```python
from build123d import *

# Parameters (mm, degrees)
SKETCH_1_W          = 126.4
SKETCH_1_H          = 68.4
SKETCH_1_W_2        = 124
SKETCH_1_H_2        = 66
EXTRUDE_1_DEPTH     = 40
SKETCH_2_W          = 126.4
SKETCH_2_H          = 68.4
EXTRUDE_1_2_DEPTH   = 1.2
CUT_EXTRUDE_1_DEPTH = 32
CUT_EXTRUDE_2_REACH = 84.243
CUT_EXTRUDE_3_DEPTH = 32
CUT_EXTRUDE_4_REACH = 103.355
CUT_EXTRUDE_5_REACH = 103.355
SKETCH_8_W          = 10
SKETCH_8_H          = 2
SKETCH_8_W_2        = 10.194480457
EXTRUDE_2_DEPTH     = 2
FILLET_1_R          = 2
CUT_EXTRUDE_6_REACH = 139.431
SKETCH_9_W          = 16
SKETCH_9_H          = 1
CUT_EXTRUDE_7_REACH = 104.715
SKETCH_10_W         = 1
SKETCH_10_H         = 16


with BuildPart() as part:
    # Эскиз1 → Extrude 1 (new body)
    with BuildSketch(Plane.XY):
        Rectangle(SKETCH_1_W, SKETCH_1_H)
        Rectangle(SKETCH_1_W_2, SKETCH_1_H_2, mode=Mode.SUBTRACT)
    extrude(amount=EXTRUDE_1_DEPTH)

    # Эскиз2 → Extrude 1 2 (add)
    with BuildSketch(Plane.XY.offset(40)):
        Rectangle(SKETCH_2_W, SKETCH_2_H)
    extrude(amount=-EXTRUDE_1_2_DEPTH)

    # Эскиз3 → Вырез-Вытянуть1 (cut)
    with BuildSketch(Plane.XY.offset(40)):
        with BuildLine():
            Line((59.2, -14), (69.2, -14))
            Line((69.2, -14), (69.2, 14))
            Line((69.2, 14), (59.2, 14))
            ThreePointArc((59.2, 14), (57.785786438, 13.414213562), (57.2, 12))
            Line((57.2, 12), (57.2, -12))
            ThreePointArc((57.2, -12), (57.785786438, -13.414213562), (59.2, -14))
        make_face()
    extrude(amount=-CUT_EXTRUDE_1_DEPTH, mode=Mode.SUBTRACT)

    # Эскиз4 → Вырез-Вытянуть2 (cut, up to next)
    with BuildSketch(Plane.XY.offset(40), mode=Mode.PRIVATE) as cut_extrude_2_sk1:
        with BuildLine():
            Line((51.2, -26), (51.2, 26))
            ThreePointArc((51.2, 26), (53.2, 28), (55.2, 26))
            Line((55.2, 26), (55.2, -26))
            ThreePointArc((55.2, -26), (53.2, -28), (51.2, -26))
        make_face()
    cut_extrude_2_tool1 = extrude(cut_extrude_2_sk1.sketch, amount=-CUT_EXTRUDE_2_REACH, mode=Mode.PRIVATE) & part.part
    # Эскиз4 → Вырез-Вытянуть2 (cut, up to next)
    with BuildSketch(Plane.XY.offset(40), mode=Mode.PRIVATE) as cut_extrude_2_sk2:
        with BuildLine():
            Line((41.2, -26), (41.2, 26))
            ThreePointArc((41.2, 26), (43.2, 28), (45.2, 26))
            Line((45.2, 26), (45.2, -26))
            ThreePointArc((45.2, -26), (43.2, -28), (41.2, -26))
        make_face()
    cut_extrude_2_tool2 = extrude(cut_extrude_2_sk2.sketch, amount=-CUT_EXTRUDE_2_REACH, mode=Mode.PRIVATE) & part.part
    # Эскиз4 → Вырез-Вытянуть2 (cut, up to next)
    with BuildSketch(Plane.XY.offset(40), mode=Mode.PRIVATE) as cut_extrude_2_sk3:
        with BuildLine():
            Line((31.2, -26), (31.2, 26))
            ThreePointArc((31.2, 26), (33.2, 28), (35.2, 26))
            Line((35.2, 26), (35.2, -26))
            ThreePointArc((35.2, -26), (33.2, -28), (31.2, -26))
        make_face()
    cut_extrude_2_tool3 = extrude(cut_extrude_2_sk3.sketch, amount=-CUT_EXTRUDE_2_REACH, mode=Mode.PRIVATE) & part.part
    # Эскиз4 → Вырез-Вытянуть2 (cut, up to next)
    with BuildSketch(Plane.XY.offset(40), mode=Mode.PRIVATE) as cut_extrude_2_sk4:
        with BuildLine():
            Line((21.2, -26), (21.2, 26))
            ThreePointArc((21.2, 26), (23.2, 28), (25.2, 26))
            Line((25.2, 26), (25.2, -26))
            ThreePointArc((25.2, -26), (23.2, -28), (21.2, -26))
        make_face()
    cut_extrude_2_tool4 = extrude(cut_extrude_2_sk4.sketch, amount=-CUT_EXTRUDE_2_REACH, mode=Mode.PRIVATE) & part.part
    # Эскиз4 → Вырез-Вытянуть2 (cut, up to next)
    with BuildSketch(Plane.XY.offset(40), mode=Mode.PRIVATE) as cut_extrude_2_sk5:
        with BuildLine():
            Line((11.2, -26), (11.2, 26))
            ThreePointArc((11.2, 26), (13.2, 28), (15.2, 26))
            Line((15.2, 26), (15.2, -26))
            ThreePointArc((15.2, -26), (13.2, -28), (11.2, -26))
        make_face()
    cut_extrude_2_tool5 = extrude(cut_extrude_2_sk5.sketch, amount=-CUT_EXTRUDE_2_REACH, mode=Mode.PRIVATE) & part.part
    # Эскиз4 → Вырез-Вытянуть2 (cut, up to next)
    with BuildSketch(Plane.XY.offset(40), mode=Mode.PRIVATE) as cut_extrude_2_sk6:
        with BuildLine():
            Line((1.2, -26), (1.2, 26))
            ThreePointArc((1.2, 26), (3.2, 28), (5.2, 26))
            Line((5.2, 26), (5.2, -26))
            ThreePointArc((5.2, -26), (3.2, -28), (1.2, -26))
        make_face()
    cut_extrude_2_tool6 = extrude(cut_extrude_2_sk6.sketch, amount=-CUT_EXTRUDE_2_REACH, mode=Mode.PRIVATE) & part.part
    # Эскиз4 → Вырез-Вытянуть2 (cut, up to next)
    with BuildSketch(Plane.XY.offset(40), mode=Mode.PRIVATE) as cut_extrude_2_sk7:
        with BuildLine():
            Line((-8.8, -26), (-8.8, 26))
            ThreePointArc((-8.8, 26), (-6.8, 28), (-4.8, 26))
            Line((-4.8, 26), (-4.8, -26))
            ThreePointArc((-4.8, -26), (-6.8, -28), (-8.8, -26))
        make_face()
    cut_extrude_2_tool7 = extrude(cut_extrude_2_sk7.sketch, amount=-CUT_EXTRUDE_2_REACH, mode=Mode.PRIVATE) & part.part
    # Эскиз4 → Вырез-Вытянуть2 (cut, up to next)
    with BuildSketch(Plane.XY.offset(40), mode=Mode.PRIVATE) as cut_extrude_2_sk8:
        with BuildLine():
            Line((-18.8, -26), (-18.8, 26))
            ThreePointArc((-18.8, 26), (-16.8, 28), (-14.8, 26))
            Line((-14.8, 26), (-14.8, -26))
            ThreePointArc((-14.8, -26), (-16.8, -28), (-18.8, -26))
        make_face()
    cut_extrude_2_tool8 = extrude(cut_extrude_2_sk8.sketch, amount=-CUT_EXTRUDE_2_REACH, mode=Mode.PRIVATE) & part.part
    # Эскиз4 → Вырез-Вытянуть2 (cut, up to next)
    with BuildSketch(Plane.XY.offset(40), mode=Mode.PRIVATE) as cut_extrude_2_sk9:
        with BuildLine():
            Line((-28.8, -26), (-28.8, 26))
            ThreePointArc((-28.8, 26), (-26.8, 28), (-24.8, 26))
            Line((-24.8, 26), (-24.8, -26))
            ThreePointArc((-24.8, -26), (-26.8, -28), (-28.8, -26))
        make_face()
    cut_extrude_2_tool9 = extrude(cut_extrude_2_sk9.sketch, amount=-CUT_EXTRUDE_2_REACH, mode=Mode.PRIVATE) & part.part
    # Эскиз4 → Вырез-Вытянуть2 (cut, up to next)
    with BuildSketch(Plane.XY.offset(40), mode=Mode.PRIVATE) as cut_extrude_2_sk10:
        with BuildLine():
            Line((-40.127823637, -29.1), (-40.127823637, -5.1))
            ThreePointArc((-40.127823637, -5.1), (-38.127823637, -3.1), (-36.127823637, -5.1))
            Line((-36.127823637, -5.1), (-36.127823637, -29.1))
            ThreePointArc((-36.127823637, -29.1), (-38.127823637, -31.1), (-40.127823637, -29.1))
        make_face()
    cut_extrude_2_tool10 = extrude(cut_extrude_2_sk10.sketch, amount=-CUT_EXTRUDE_2_REACH, mode=Mode.PRIVATE) & part.part
    # Эскиз4 → Вырез-Вытянуть2 (cut, up to next)
    with BuildSketch(Plane.XY.offset(40), mode=Mode.PRIVATE) as cut_extrude_2_sk11:
        with BuildLine():
            Line((-46.127823637, -29.1), (-46.127823637, -5.1))
            ThreePointArc((-46.127823637, -5.1), (-44.127823637, -3.1), (-42.127823637, -5.1))
            Line((-42.127823637, -5.1), (-42.127823637, -29.1))
            ThreePointArc((-42.127823637, -29.1), (-44.127823637, -31.1), (-46.127823637, -29.1))
        make_face()
    cut_extrude_2_tool11 = extrude(cut_extrude_2_sk11.sketch, amount=-CUT_EXTRUDE_2_REACH, mode=Mode.PRIVATE) & part.part
    # Эскиз4 → Вырез-Вытянуть2 (cut, up to next)
    with BuildSketch(Plane.XY.offset(40), mode=Mode.PRIVATE) as cut_extrude_2_sk12:
        with BuildLine():
            Line((-52.127823637, -29.1), (-52.127823637, -5.1))
            ThreePointArc((-52.127823637, -5.1), (-50.127823637, -3.1), (-48.127823637, -5.1))
            Line((-48.127823637, -5.1), (-48.127823637, -29.1))
            ThreePointArc((-48.127823637, -29.1), (-50.127823637, -31.1), (-52.127823637, -29.1))
        make_face()
    cut_extrude_2_tool12 = extrude(cut_extrude_2_sk12.sketch, amount=-CUT_EXTRUDE_2_REACH, mode=Mode.PRIVATE) & part.part
    # Эскиз4 → Вырез-Вытянуть2 (cut, up to next)
    with BuildSketch(Plane.XY.offset(40), mode=Mode.PRIVATE) as cut_extrude_2_sk13:
        with BuildLine():
            Line((-58.127823637, -29.1), (-58.127823637, -5.1))
            ThreePointArc((-58.127823637, -5.1), (-56.127823637, -3.1), (-54.127823637, -5.1))
            Line((-54.127823637, -5.1), (-54.127823637, -29.1))
            ThreePointArc((-54.127823637, -29.1), (-56.127823637, -31.1), (-58.127823637, -29.1))
        make_face()
    cut_extrude_2_tool13 = extrude(cut_extrude_2_sk13.sketch, amount=-CUT_EXTRUDE_2_REACH, mode=Mode.PRIVATE) & part.part
    add(cut_extrude_2_tool1.solids().sort_by_distance((53.2, 0, 40))[0], mode=Mode.SUBTRACT)
    add(cut_extrude_2_tool2.solids().sort_by_distance((43.2, 0, 40))[0], mode=Mode.SUBTRACT)
    add(cut_extrude_2_tool3.solids().sort_by_distance((33.2, 0, 40))[0], mode=Mode.SUBTRACT)
    add(cut_extrude_2_tool4.solids().sort_by_distance((23.2, 0, 40))[0], mode=Mode.SUBTRACT)
    add(cut_extrude_2_tool5.solids().sort_by_distance((13.2, 0, 40))[0], mode=Mode.SUBTRACT)
    add(cut_extrude_2_tool6.solids().sort_by_distance((3.2, 0, 40))[0], mode=Mode.SUBTRACT)
    add(cut_extrude_2_tool7.solids().sort_by_distance((-6.8, 0, 40))[0], mode=Mode.SUBTRACT)
    add(cut_extrude_2_tool8.solids().sort_by_distance((-16.8, 0, 40))[0], mode=Mode.SUBTRACT)
    add(cut_extrude_2_tool9.solids().sort_by_distance((-26.8, 0, 40))[0], mode=Mode.SUBTRACT)
    add(cut_extrude_2_tool10.solids().sort_by_distance((-38.127824, -17.1, 40))[0], mode=Mode.SUBTRACT)
    add(cut_extrude_2_tool11.solids().sort_by_distance((-44.127824, -17.1, 40))[0], mode=Mode.SUBTRACT)
    add(cut_extrude_2_tool12.solids().sort_by_distance((-50.127824, -17.1, 40))[0], mode=Mode.SUBTRACT)
    add(cut_extrude_2_tool13.solids().sort_by_distance((-56.127824, -17.1, 40))[0], mode=Mode.SUBTRACT)

    # Эскиз5 → Вырез-Вытянуть3 (cut)
    with BuildSketch(Plane.XY.offset(40)):
        with BuildLine():
            Line((-59.2, 48.521499027), (-35.2, 48.521499027))
            Line((-35.2, 48.521499027), (-35.2, 21.878500973))
            ThreePointArc((-35.2, 21.878500973), (-35.785786438, 20.46428741), (-37.2, 19.878500973))
            Line((-37.2, 19.878500973), (-57.2, 19.878500973))
            ThreePointArc((-57.2, 19.878500973), (-58.614213562, 20.46428741), (-59.2, 21.878500973))
            Line((-59.2, 21.878500973), (-59.2, 48.521499027))
        make_face()
    extrude(amount=-CUT_EXTRUDE_3_DEPTH, mode=Mode.SUBTRACT)

    # Эскиз6 → Вырез-Вытянуть4 (cut, up to next)
    with BuildSketch(Plane.XZ.offset(34.2), mode=Mode.PRIVATE) as cut_extrude_4_sk1:
        with BuildLine():
            Line((53.2, 0), (-43.2, 0))
            Line((-43.2, 0), (-43.2, 26))
            ThreePointArc((-43.2, 26), (-42.614213562, 27.414213562), (-41.2, 28))
            Line((-41.2, 28), (51.2, 28))
            ThreePointArc((51.2, 28), (52.614213562, 27.414213562), (53.2, 26))
            Line((53.2, 26), (53.2, 0))
        make_face()
    cut_extrude_4_tool1 = extrude(cut_extrude_4_sk1.sketch, amount=-CUT_EXTRUDE_4_REACH, mode=Mode.PRIVATE) & part.part
    add(cut_extrude_4_tool1.solids().sort_by_distance((5, -34.2, 13.991374))[0], mode=Mode.SUBTRACT)

    # Эскиз7 → Вырез-Вытянуть5 (cut, up to next)
    with BuildSketch(Plane(origin=(0, 34.2, 0), x_dir=(1, 0, 0), z_dir=(0, 1, 0)), mode=Mode.PRIVATE) as cut_extrude_5_sk1:
        with BuildLine():
            Line((53.2, 0), (-25.2, 0))
            Line((-25.2, 0), (-25.2, -26))
            ThreePointArc((-25.2, -26), (-24.614213562, -27.414213562), (-23.2, -28))
            Line((-23.2, -28), (51.2, -28))
            ThreePointArc((51.2, -28), (52.614213562, -27.414213562), (53.2, -26))
            Line((53.2, -26), (53.2, 0))
        make_face()
    cut_extrude_5_tool1 = extrude(cut_extrude_5_sk1.sketch, amount=-CUT_EXTRUDE_5_REACH, mode=Mode.PRIVATE) & part.part
    add(cut_extrude_5_tool1.solids().sort_by_distance((14, 34.2, 13.989392))[0], mode=Mode.SUBTRACT)

    # Эскиз8 → Бобышка-Вытянуть2 (add)
    with BuildSketch(Plane(origin=(0, 0, 0), x_dir=(-1, 0, 0), z_dir=(0, 0, -1))):
        with Locations((-58.2, 35.2)):
            Rectangle(SKETCH_8_W, SKETCH_8_H)
        with Locations((-58.2, -35.2)):
            Rectangle(SKETCH_8_W, SKETCH_8_H)
        with Locations((58.102759772, 35.2)):
            Rectangle(SKETCH_8_W_2, SKETCH_8_H)
        with Locations((58.102759772, -35.2)):
            Rectangle(SKETCH_8_W_2, SKETCH_8_H)
    extrude(amount=-EXTRUDE_2_DEPTH)

    # Скругление1
    fillet_1_edges = [part.edges().sort_by_distance(p)[0] for p in [
        (-58.102759771, -34.2, 2),
        (58.2, -34.2, 2),
        (58.2, 34.2, 2),
        (-58.102759771, 34.2, 2),
    ]]
    fillet(fillet_1_edges, radius=FILLET_1_R - 0.0001)  # a hair under: the kernel refuses the full size

    # Эскиз9 → Вырез-Вытянуть6 (cut, up to next)
    with BuildSketch(Plane(origin=(63.2, 0, 0), x_dir=(0, 0, -1), z_dir=(1, 0, 0)), mode=Mode.PRIVATE) as cut_extrude_6_sk1:
        Rectangle(SKETCH_9_W, SKETCH_9_H)
    cut_extrude_6_tool1 = extrude(cut_extrude_6_sk1.sketch, amount=-CUT_EXTRUDE_6_REACH, mode=Mode.PRIVATE) & part.part
    add(cut_extrude_6_tool1.solids().sort_by_distance((63.2, 0, 0))[0], mode=Mode.SUBTRACT)

    # Эскиз10 → Вырез-Вытянуть7 (cut, up to next)
    with BuildSketch(Plane(origin=(0, 34.2, 0), x_dir=(1, 0, 0), z_dir=(0, 1, 0)), mode=Mode.PRIVATE) as cut_extrude_7_sk1:
        with Locations((-44.530737739, 0)):
            Rectangle(SKETCH_10_W, SKETCH_10_H)
    cut_extrude_7_tool1 = extrude(cut_extrude_7_sk1.sketch, amount=-CUT_EXTRUDE_7_REACH, mode=Mode.PRIVATE) & part.part
    add(cut_extrude_7_tool1.solids().sort_by_distance((-44.530738, 34.2, 0))[0], mode=Mode.SUBTRACT)


solid = part.part
```
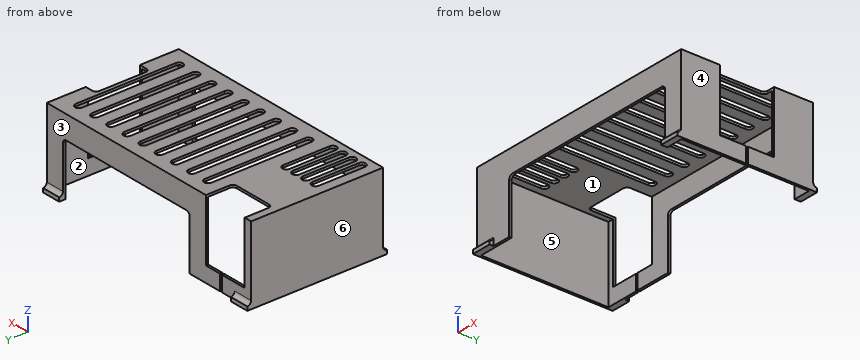
Design review of the part built by this model. Coordinates are the model's own, in mm. Face numbers are marked on the shaded views. A direction names the side the tool comes from. Give positions to 0.01 mm unless a question says otherwise; leave off trailing zeros. Write each loop counter-clockwise with the first axis right and the second up, starting at its lowest first coordinate (ties: lowest second). Pieces come first, ordered by that corner, then holes. Notation, with made-up numbers: (14.5, 29) -> (20.5, 29) arc R38 ccw to (20.5, 68) -> close; hole circle Ø5 at (-4, 27.25). An arc over 180 degrees is marked (long way). Answer in a Markdown table with one row per item.
(1) For the marked faces 5 and 6, list the 3-axis set-ups (+Z, -Z, +X, -X, +Y, -Y) from which the entire face can be reached by the end or side of a thin tool; tool diameter is ignored.
Results:
| item | result |
|---|---|
| face 5 | -Z |
| face 6 | +Z, -Z, -X, +Y, -Y |
(2) Mouldability with a two-part tool opening along Y and no side actions: class the marked faces 1, 2, 3 and 4 as +Y half, -Y half, draft (parallel to the pull), parting line (faces both ways), or undercut.
Results:
| item | result |
|---|---|
| face 1 | undercut |
| face 2 | undercut |
| face 3 | +Y half |
| face 4 | draft |
(3) Consider section C-C (x = 13.2). State the section outline as (y, z) points, then the cut area to 3 significant figures.
Results:
| item | result |
|---|---|
| outline | (-34.2, 28) -> (-33, 28) -> (-33, 38.8) -> (-28, 38.8) -> (-28, 40) -> (-34.2, 40) -> close; (28, 38.8) -> (33, 38.8) -> (33, 28) -> (34.2, 28) -> (34.2, 40) -> (28, 40) -> close |
| area | 40.8 mm2 |
(4) Consider section A-A (z = 22). State the section outline as (x, y) points.
Results:
| item | result |
|---|---|
| outline | (-63.2, -34.2) -> (-43.2, -34.2) -> (-43.2, -33) -> (-62, -33) -> (-62, 33) -> (-59.2, 33) -> (-59.2, 34.2) -> (-63.2, 34.2) -> close; (-35.2, 33) -> (-25.2, 33) -> (-25.2, 34.2) -> (-35.2, 34.2) -> close; (53.2, -34.2) -> (63.2, -34.2) -> (63.2, -14) -> (62, -14) -> (62, -33) -> (53.2, -33) -> close; (53.2, 33) -> (62, 33) -> (62, 14) -> (63.2, 14) -> (63.2, 34.2) -> (53.2, 34.2) -> close |
(5) Clearance check with flat-ended pins moving along their axes: pin 1 (1.3 mm diameter, centred on y = 1, z = 39.5, fed in from +X); pin 2 (5 mm diameter, centred on x = -24, y = -4.5, fed in from -Z); pin 3 (1 mm diameter, centred on y = -4.5, z = 21, fed in from +X). State where each tip first meets the part, or that it passes through.
Results:
| item | result |
|---|---|
| pin 1 | x = 57.2 |
| pin 2 | z = 38.8 |
| pin 3 | x = -62 |
(6) To check wall thickness, follow probe 1 along X at (y, z) = (-19.5, 21); probe 2 along Z at (x, y) = (31.5, 29.5); probe 3 along Y at (x, z) = (26, 38). State the ranges of each line that lie inside material, in increasing order.
Results:
| item | result |
|---|---|
| probe 1 | -63.2 to -62, 62 to 63.2 |
| probe 2 | 38.8 to 40 |
| probe 3 | -34.2 to -33, 33 to 34.2 |
(7) Consider section D-D (y = 17). Count the separate pieces of the cut face and the enclosed holes in it, then the cut area to 3 significant figures.
Results:
| item | result |
|---|---|
| separate pieces | 10 |
| enclosed holes | 0 |
| area | 202 mm2 |
(8) Consider section B-B (y = 29.5). State the section outline as (x, z) points, then the cut area to 3 significant figures.
Results:
| item | result |
|---|---|
| outline | (-63.2, 0) -> (-62, 0) -> (-62, 38.8) -> (-59.2, 38.8) -> (-59.2, 40) -> (-63.2, 40) -> close; (-35.2, 38.8) -> (62, 38.8) -> (62, 0) -> (63.2, 0) -> (63.2, 40) -> (-35.2, 40) -> close |
| area | 216 mm2 |
